Can you work these out from the model? Positions are in its coordinate system, mm. Coordinates: 2 decimals unless noted, no trailing zeros. Loops run counter-clockwise (first coordinate to the right, second up) from the corner with the lowest first, then second, coordinate; pieces in that order, holes last. Notation, with made-up numbers: M 63.25,49 L 88.25,49 A12 cw 88.25,62 Z; hole C 72,58.25 d3. An arc over 180 degrees is marked long. Answer as a JSON object with one key per item and string values. Group by question number.
Item 1: Suppose I cut it at C-C (z = 0.4). Write out the boundary of the cut face in (x, y), then the cut area to 3 significant figures.
Item 2: If I drill on line 1 (Y direction, x = -4, z = 0.45); line 2 (Y direction, x = -32.5, z = 0.25); line 3 (X direction, y = -27, z = 1.35), over which ranges is the centre line in solid material (lowest first)?
Item 3: I'm going to push flat-ended pins straight in: pin 1 Ø2 at (x, y) = (-12.5, -15) entering from -Z; pin 2 Ø1 at (y, z) = (2.5, 0.5) entering from +X; pin 3 Ø1 at (y, z) = (-8, 0.5) entering from +X. Where does each tip first touch, or does it pass through?
Item 4: Suppose I cut it at D-D (x = -16.5). Write out the boundary of the cut face in (y, z), then the cut area to 3 significant figures.
Item 5: Suppose I cut it at B-B (x = -32). Write out the boundary of the cut face in (y, z), then the cut area to 3 significant figures.
Item 6: Suppose I cut it at A-A (y = -27.5). Write out the boundary of the cut face in (x, z), then the cut area to 3 significant figures.
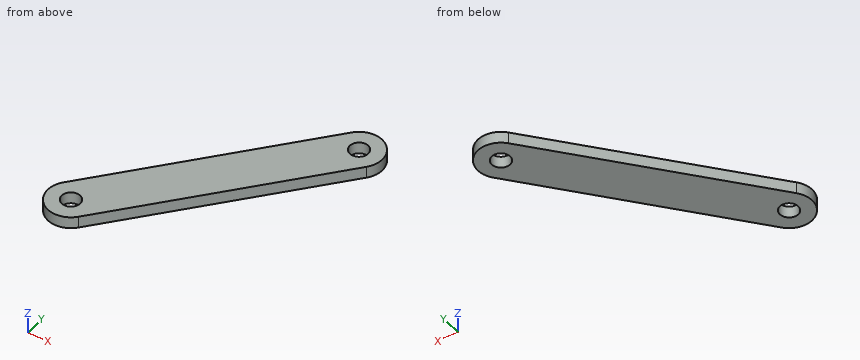
Autodesk Inventor part; units mm, degrees
ref_plane "YZ Plane" through (0, 0, 0) normal (1, 0, 0) x (0, 1, 0)
ref_plane "XZ Plane" through (0, 0, 0) normal (0, 1, 0) x (-1, 0, 0)
ref_plane "XY Plane" through (0, 0, 0) normal (0, 0, 1) x (1, 0, 0)
sketch "Sketch1" plane through (0, 0, 0) normal (0, 0, 1) x (1, 0, 0)
  circle A0 centre (-5.1902, 4.697) radius 1.6
  circle A1 centre (-32.4398, -28.1035) radius 1.6
  line L0 (-32.4398, -28.1035) -> (-5.1902, 4.697) construction
  line L1 (-29.363, -30.6596) -> (-2.1134, 2.1409)
  line L2 (-8.267, 7.2531) -> (-35.5166, -25.5474)
  arc A2 (-35.5166, -25.5474) -> (-29.363, -30.6596) centre (-32.4398, -28.1035) ccw
  arc A3 (-2.1134, 2.1409) -> (-8.267, 7.2531) centre (-5.1902, 4.697) ccw
  point P0 (0, 0)
  point P1 (-18.815, -11.7033)
  dimension "d0" = 4
extrude "Extrusion1" add sketch "Sketch1" along normal blind 2
properties part number "linkage-arm"
From the geometry:
{
 "1": {"outline": "M -35.52,-25.55 A4 ccw -29.36,-30.66 L -2.11,2.14 A4 ccw -8.27,7.25 Z; hole C -32.44,-28.1 d3.2; hole C -5.19,4.7 d3.2", "area": "375 mm2"},
 "2": {"line 1": "-0.13 to 3.63, 5.77 to 8.52", "line 2": "-32.1 to -29.7, -26.5 to -21.92", "line 3": "-36.28 to -33.6, -31.28 to -26.32"},
 "3": {"pin 1": "through", "pin 2": "x = -1.57", "pin 3": "x = -10.12"},
 "4": {"outline": "M -15.18,0 L -2.66,0 L -2.66,2 L -15.18,2 Z", "area": "25.0 mm2"},
 "5": {"outline": "M -32.08,0 L -29.64,0 L -29.64,2 L -32.08,2 Z; M -26.57,0 L -21.31,0 L -21.31,2 L -26.57,2 Z", "area": "15.4 mm2"},
 "6": {"outline": "M -36.39,0 L -33.92,0 L -33.92,2 L -36.39,2 Z; M -30.96,0 L -26.74,0 L -26.74,2 L -30.96,2 Z", "area": "13.4 mm2"}
}
